Design review of the part built by this model. Coordinates are the model's own, in mm. A direction names the side the tool comes from. Coordinates: 2 decimals unless noted, no trailing zeros. Loops run counter-clockwise (first coordinate to the right, second up) from the corner with the lowest first, then second, coordinate; pieces in that order, holes last. Notation, with made-up numbers: (33.5, -36.5) - (91.5, -36.5) arc R18 cw to (91.5, -7.5) - close; hole circle Ø8 at (45.25, 17). An arc over 180 degrees is marked (long way). One line per question, with ' | ' between items.
from build123d import *

# Parameters (mm, degrees)
F1_DEPTH = 61
F2_W     = 25
F2_H     = 21
F3_DEPTH = 4
F4_R     = 1.75
F5_DEPTH = 18


with BuildPart() as f1:
    # F0 (on Top) → F1 (new body)
    with BuildSketch(Plane.XY):
        with BuildLine():
            Line((-9.5, -0.15), (-9.5, 8.35))
            ThreePointArc((-9.5, 8.35), (-6.543126, 14.742744), (0, 17.35))
            Line((0, 17.35), (0, 17.85))
            ThreePointArc((0, 17.85), (-3.721623, 17.523131), (-7.329289, 16.552532))
            ThreePointArc((-7.329289, 16.552532), (-10.040473, 12.843207), (-11, 8.35))
            Line((-11, 8.35), (-11, 1.35))
            Line((-11, 1.35), (-17.922894, 1.35))
            Line((-17.922894, 1.35), (-17.922894, -4.709674))
            Line((-17.922894, -4.709674), (-20.105763, -10.681977))
            Line((-20.105763, -10.681977), (-9.422894, -9.459674))
            Line((-9.422894, -9.459674), (0, -9.459674))
            Line((0, -9.459674), (0, -6.65))
            Line((0, -6.65), (-5.4, -6.65))
            ThreePointArc((-5.4, -6.65), (-6, -6.027996), (-6.6, -6.65))
            Line((-6.6, -6.65), (-15.478196, -6.65))
            Line((-15.478196, -6.65), (-15.478196, -4.39619))
            ThreePointArc((-15.478196, -4.39619), (-14.565471, -3.389066), (-15.5, -2.402142))
            Line((-15.5, -2.402142), (-15.5, -0.15))
            Line((-15.5, -0.15), (-12.85729, -0.15))
            ThreePointArc((-12.85729, -0.15), (-12.25729, -0.75), (-11.65729, -0.15))
            Line((-11.65729, -0.15), (-9.5, -0.15))
        make_face()
        with BuildLine():
            Line((0, 17.85), (0, 17.35))
            ThreePointArc((0, 17.35), (6.543126, 14.742744), (9.5, 8.35))
            Line((9.5, 8.35), (9.5, -0.15))
            Line((9.5, -0.15), (11.65729, -0.15))
            ThreePointArc((11.65729, -0.15), (12.25729, -0.75), (12.85729, -0.15))
            Line((12.85729, -0.15), (15.5, -0.15))
            Line((15.5, -0.15), (15.5, -2.402142))
            ThreePointArc((15.5, -2.402142), (14.565471, -3.389066), (15.478196, -4.39619))
            Line((15.478196, -4.39619), (15.478196, -6.65))
            Line((15.478196, -6.65), (6.6, -6.65))
            ThreePointArc((6.6, -6.65), (6, -6.027996), (5.4, -6.65))
            Line((5.4, -6.65), (0, -6.65))
            Line((0, -6.65), (0, -9.459674))
            Line((0, -9.459674), (9.422894, -9.459674))
            Line((9.422894, -9.459674), (20.105763, -10.681977))
            Line((20.105763, -10.681977), (17.922894, -4.709674))
            Line((17.922894, -4.709674), (17.922894, 1.35))
            Line((17.922894, 1.35), (11, 1.35))
            Line((11, 1.35), (11, 8.35))
            ThreePointArc((11, 8.35), (10.040473, 12.843207), (7.329289, 16.552532))
            ThreePointArc((7.329289, 16.552532), (3.721623, 17.523131), (0, 17.85))
        make_face()
    extrude(amount=F1_DEPTH)

    # F2 (on face) → F3 (cut, symmetric)
    with BuildSketch(Plane.XZ.offset(9.459674)):
        with Locations((0, 50.5)):
            Rectangle(F2_W, F2_H)
    extrude(amount=F3_DEPTH, both=True, mode=Mode.SUBTRACT)

    # F4 (on face) → F5 (join)
    with BuildSketch(Plane.XY.offset(61)):
        with Locations((-15.565411, -3.4)):
            Circle(F4_R)
        with Locations((15.565411, -3.4)):
            Circle(F4_R)
    extrude(amount=-F5_DEPTH)


solid = f1.part
Q1. Take a section at C-C (x = -2). Give the boundary of the cut face in (y, z), plus the area to 3 significant figures.
Returned:
outline: (-9.46, 0) - (-6.65, 0) - (-6.65, 40) - (-9.46, 40) - close; (17.14, 0) - (17.76, 0) - (17.76, 61) - (17.14, 61) - close | area: 150 mm²
Q2. Tool access review of faces 4 (the flat face through (15.478, -6, 30)), 5 (the flat face through (-14.84, -10.08, 30.07)), 6 (the cylindrical face through (-12.27, -0.75, 30.07)): name each direction out of +Z, -Z, +X, -X, +Y, -Y from which nothing blocks a thin tool from reaching the whole face with its end or side.
Returned:
face 4: -Z | face 5: +Z, -Z, -Y | face 6: +Z, -Z
Q3. Take a section at D-D (y = -3.4). Give the boundary of the cut face in (x, z).
Returned:
outline: (-17.92, 0) - (-14.57, 0) - (-14.57, 43) - (-13.82, 43) - (-13.82, 61) - (-17.92, 61) - close; (13.82, 43) - (14.57, 43) - (14.57, 0) - (17.92, 0) - (17.92, 61) - (13.82, 61) - close
Q4. Draft analysis for pull direction X (two halves, no side actions). For faces 1 (the flat face through (14.3, -3.4, 43)), 2 (the flat face through (-14, 1.35, 30)), 3 (the cylindrical face through (-10.014, 12.902, 30.073)), state which applies: +X half, -X half, draft (parallel to the pull), parting line (faces both ways), or undercut.
Returned:
face 1: undercut | face 2: draft | face 3: -X half
Q5. Take a section at A-A (y = 5.5). Give the boundary of the cut face in (x, z).
Returned:
outline: (-11, 0) - (-9.5, 0) - (-9.5, 61) - (-11, 61) - close; (9.5, 0) - (11, 0) - (11, 61) - (9.5, 61) - close
Q6. For pin 1 (3.5 mm diameter, centred on y = 4, z = 31, fed in from -X); pin 2 (4 mm diameter, centred on x = 11, y = -3, fed in from +Z); pin 3 (10 mm diameter, centred on x = 10.5, z = 20.5, fed in from +Y); pin 4 (0.9 mm diameter, centred on y = -8.5, z = 47.5, fed in from +X), all flat-tipped, find the tip position at first contact; note any pin that passes through.
Returned:
pin 1: stops at x = -11 | pin 2: passes through | pin 3: stops at y = 17.13 | pin 4: stops at x = 19.47
Q7. To check wall thickness, follow line 1 along X through (y, z) = (3.25, 32.5); line 2 along X through (y, z) = (0.5, 33); line 3 along X through (y, z) = (-6.5, 37). State the ranges of each line that lie inside material, in increasing order.
Returned:
line 1: x = -11 to -9.5, 9.5 to 11 | line 2: x = -17.92 to -9.5, 9.5 to 17.92 | line 3: x = -18.58 to -15.48, -6.59 to -5.41, 5.41 to 6.59, 15.48 to 18.58
